Can you work these out from the model? Positions are in its coordinate system, mm. A direction names the side the tool comes from. Round coordinates to 2 decimals unless told otherwise and drop trailing zeros. Write each loop counter-clockwise with the first axis right and the second up, starting at its lowest first coordinate (ties: lowest second). Pieces come first, ordered by that corner, then holes. Notation, with made-up numbers: M 38.5,1 L 48.5,1 A33 cw 48.5,36 Z; hole C 74.25,82.25 d4. An arc over 180 degrees is marked long. Answer as a JSON object with one key per item and string values. Group by question number.
1) Suppose I cut it at B-B, the plane y = 19. Write out the boundary of the cut face in (x, z), and give its area (4 significant figures).
2) On a 3-axis mill with a long thin cutter (end or side, diameter ignored), from which of +Z, -Z, +X, -X, +Y, -Y can I reach the whole of each face in a straight line? I mean faces 1 (the flat face through (-1, 13.05, 5)), 2 (the cylindrical face through (9.95, -7.46, 7.71)). Say none if no direction works.
3) Suppose I cut it at A-A, the plane x = 24.9. Write out the boundary of the cut face in (y, z) (3 decimals).
4) If we mould it in two halves opening along Z, with no side actions, what happens to faces 3 (the flat face through (-13, -7, 4.5)), 4 (the cylindrical face through (-4.85, 10.24, 4.59)), 5 (the cylindrical face through (27.76, -7.46, 2.72))? For each: +Z half, -Z half, draft (parallel to the pull), parting line (faces both ways), or undercut.
5) Suppose I cut it at C-C, the plane x = 2.5. Write out the boundary of the cut face in (y, z), and give its area (4 significant figures).
6) Please list where these lines run through material, in increasing order: L1, parallel to Y at x = -23.1, z = 4.5; L2, parallel to X at y = 18, z = 2.25. Write a range as [from, to].
7) I'm going to push flat-ended pins straight in: pin 1 Ø2.5 at (x, y) = (-12.5, -8) entering from +Z; pin 2 Ø1.5 at (x, z) = (13, -0.5) entering from +Y; pin 3 Ø3 at (x, y) = (-2.1, 10.3) entering from +Z. Where does each tip first touch, or does it pass through?
Autodesk Inventor part; units mm, degrees
ref_plane "YZ Plane" through (0, 0, 0) normal (1, 0, 0) x (0, 1, 0)
ref_plane "XZ Plane" through (0, 0, 0) normal (0, 1, 0) x (-1, 0, 0)
ref_plane "XY Plane" through (0, 0, 0) normal (0, 0, 1) x (1, 0, 0)
sketch "Sketch1" plane through (0, 0, 0) normal (0, 0, 1) x (1, 0, 0)
  line L0 (0, 0) -> (-25, 0)
  line L1 (-25, 25) -> (0, 25)
  line L2 (0, 25) -> (0, 0)
  circle A0 centre (-23.1, 22.7984) radius 1.1
  circle A1 centre (-2.1, 22.8) radius 1.1
  circle A2 centre (-23.1, 10.2984) radius 1.1
  circle A3 centre (-2.1, 10.3) radius 1.1
  line L3 (-25, 0) -> (-25.2, 0)
  line L4 (-25.2, 0) -> (-25.2, 25)
  line L5 (-25.2, 25) -> (-25, 25)
  dimension "d2" = 2.2
  dimension "d5" = 2.2
  dimension "d7" = 12.5
  dimension "d8" = 2.2
  dimension "d9" = 2.2
  dimension "d14" = 12.5
  dimension "d31" = 2.1
  dimension "d46" = 0.2
  dimension "d47" = 2.1
  dimension "d48" = 2.1
extrude "Base" add sketch "Sketch1" along normal blind 2
sketch "Sketch2" plane through (0, 0, 2) normal (0, 0, 1) x (1, 0, 0)
  line L0 (-26.5, 0) -> (-26.5, 26.5)
  line L1 (-26.5, 26.5) -> (1.5, 26.5)
  line L2 (1.5, 26.5) -> (1.5, 0)
  line L3 (1.5, 0) -> (0, 0)
  line L4 (0, 25) -> (-25.2, 25)
  line L5 (0, 0) -> (0, 25)
  line L6 (-25.2, 25) -> (-25.2, 0)
  line L7 (-25.2, 0) -> (-26.5, 0)
  point P0 (-25, 25)
  point P1 (-25, 0)
  dimension "d16" = 26.5
  dimension "d17" = 28
extrude "Walls" add sketch "Sketch2" along normal blind 5.25 and the other way blind 2
sketch "Sketch3" plane through (0, 0, 2) normal (0, 0, 1) x (1, 0, 0)
  circle A0 centre (-23.1, 10.2984) radius 1.1
  circle A1 centre (-23.1, 10.2984) radius 1.6
  circle A2 centre (-2.1, 10.3) radius 1.1
  circle A3 centre (-2.1, 10.3) radius 1.6
  circle A4 centre (-23.1, 22.7984) radius 1.1
  circle A5 centre (-23.1, 22.7984) radius 1.6
  circle A6 centre (-2.1, 22.8) radius 1.1
  circle A7 centre (-2.1, 22.8) radius 1.6
  point P0 (0, 0)
  dimension "d22" = 3.2
  dimension "d23" = 3.2
  dimension "d24" = 3.2
  dimension "d25" = 3.2
extrude "Spacers" add sketch "Sketch3" along normal up to surface (5.25 mm away)
sketch "Sketch4" plane through (0, 0, 2) normal (0, 0, 1) x (1, 0, 0)
  circle A0 centre (-23.1, 10.2984) radius 1.1
  arc A1 (-23.1938, 7.55) -> (-23.1, 13.0484) centre (-23.1, 10.2984) ccw
  circle A2 centre (-2.1, 10.3) radius 1.1
  arc A3 (-2.1, 13.05) -> (-2.1, 7.55) centre (-2.1, 10.3) ccw
  circle A4 centre (-23.1, 22.7984) radius 1.1
  circle A5 centre (-2.1, 22.8) radius 1.1
  line L0 (-4.85, 22.8) -> (-4.85, 25)
  line L1 (-25.2, 25) -> (0, 25)
  line L2 (-2.1, 20.05) -> (0, 20.05)
  line L3 (0, 25) -> (0, 0)
  line L4 (-2.1, 13.05) -> (0, 13.05)
  line L5 (-2.1, 7.55) -> (0, 7.55)
  line L6 (-23.1, 13.0484) -> (-25.2, 13.0484)
  line L7 (-23.1938, 7.55) -> (-25, 7.55)
  arc A6 (-4.85, 22.8) -> (-2.1, 20.05) centre (-2.1, 22.8) ccw
  line L8 (-25, 7.55) -> (-25.2, 7.55)
  line L9 (-25.2, 13.0484) -> (-25.2, 13.0484)
  line L10 (-25.2, 25) -> (-25.2, 0)
  line L11 (-25.2, 20.0484) -> (-25.2, 20.0484)
  line L12 (-20.35, 22.7984) -> (-20.35, 25.6874)
  line L13 (-23.1, 20.0484) -> (-25.85, 20.0484)
  arc A7 (-23.1, 20.0484) -> (-20.35, 22.7984) centre (-23.1, 22.7984) ccw
  point P0 (-25, 25)
  point P1 (-20.35, 25)
  point P2 (-25.2, 20.0484)
  dimension "d33" = 5.5
  dimension "d34" = 5.5
extrude "Spacer blocks" add sketch "Sketch4" along normal up to surface (5.25 mm away)
sketch "Sketch5" plane through (0, 0, 0) normal (0, 0, -1) x (-1, 0, 0)
  line L0 (-1.5, 26.5) -> (-1.5, 0)
  circle A0 centre (12.4, 10.3) radius 4.5
  point P0 (0, 0)
  dimension "d39" = 13.9
  dimension "d40" = 9
extrude "Camera Hole" cut sketch "Sketch5" against normal through all
fillet "Outside Fillet - 2mm" radius 2 1 edges at (-7.9, 10.3, 0)
fillet "Inside Fillet - 1mm" radius 0.5 2 edges at (-7.9, 10.3, 1.9999) (-7.9, 10.3, 2)
chamfer "Chamfer1" distance 0.5 angle 45 5 edges at (1.5, 13.25, 0) (1.5, 26.5, 3.625) (-12.5, 26.5, 0) (-26.5, 26.5, 3.625) (-26.5, 13.25, 0)
sketch "Sketch6" plane through (-25.2, 0, 2) normal (0, -1, 0) x (1, 0, 0)
  line L0 (-0.8, -2) -> (-1.3, -1.5)
  line L1 (26.2, -2) -> (-0.8, -2)
  line L2 (26.7, -1.5) -> (26.2, -2)
  line L3 (26.7, -1.5) -> (26.7, 5.25)
  line L4 (25.2, 5.25) -> (26.7, 5.25)
  line L5 (25.2, 0) -> (25.2, 5.25)
  line L6 (0, 0) -> (25.2, 0)
  line L7 (0, 0) -> (0, 5.25)
  line L8 (-1.3, 5.25) -> (0, 5.25)
  line L9 (-1.3, -1.5) -> (-1.3, 5.25)
  point P0 (25.2, -2)
extrude "Bottom Extension" add sketch "Sketch6" along normal blind 5
sketch "Sketch7" plane through (-25.2, -5, 2) normal (0, -1, 0) x (1, 0, 0)
  line L0 (26.7, 5.25) -> (25.2, 5.25)
  line L1 (26.7, 5.25) -> (20.1, 5.25)
  line L2 (20.1, 5.25) -> (20.1, -2)
  line L3 (20.1, -2) -> (50.1, -2)
  line L4 (50.1, -2) -> (50.1, 5.25)
  line L5 (50.1, 5.25) -> (26.7, 5.25)
  line L6 (26.7, 5.25) -> (25.2, 5.25) construction
  line L7 (25.2, 5.25) -> (25.2, 0) construction
  line L8 (25.2, 0) -> (0, 0) construction
  line L9 (0, 0) -> (0, 5.25) construction
  line L10 (0, 5.25) -> (-1.3, 5.25) construction
  line L11 (-1.3, 5.25) -> (-1.3, -1.5) construction
  line L12 (-1.3, -1.5) -> (-0.8, -2) construction
  line L13 (-0.8, -2) -> (26.2, -2) construction
  line L14 (26.2, -2) -> (26.7, -1.5) construction
  line L15 (26.7, -1.5) -> (26.7, 5.25) construction
  line L16 (20.1, -2) -> (-0.8, -2)
  line L17 (-1.3, -1.5) -> (-0.8, -2)
  line L18 (-1.3, -1.5) -> (-1.3, 5.25)
  line L19 (-1.3, 5.25) -> (0, 5.25)
  line L20 (0, 5.25) -> (5.1, 5.25)
  line L21 (5.1, 5.25) -> (5.1, 0)
  line L22 (5.1, 0) -> (20.1, 0)
  line L23 (5.1, 0) -> (5.1, 2.5)
  line L24 (5.1, 2.5) -> (20.1, 2.5)
  point P0 (25.2, -2)
  dimension "d54" = 6.6
  dimension "d55" = 30
  dimension "d58" = 5.1
  dimension "d59" = 2.5
extrude "Mounting Arm" add sketch "Sketch7" along normal blind 5
sketch "Sketch8" plane through (-25.2, -5, 2) normal (0, 1, 0) x (1, 0, 0)
  line L0 (50.1, 2) -> (50.1, -5.25)
  circle A0 centre (50.1, -1.625) radius 15
  point P0 (25.2, 2)
  dimension "d60" = 30
extrude "Mounting Disk" add sketch "Sketch8" against normal up to surface (5 mm away)
fillet "Fillet4" radius 2.5 2 edges at (10.3446, -7.5, 0) (10.3446, -7.5, 7.25)
sketch "Sketch9" plane through (-25.2, -5, 2) normal (0, 1, 0) x (1, 0, 0)
  arc A0 (36.0488, -6.875) -> (36.0488, 3.625) centre (50.1, -1.625) ccw
  circle A1 centre (50.1, -1.625) radius 3
  point P0 (25.2, 2)
  dimension "d64" = 6
extrude "Center Hole" cut sketch "Sketch9" against normal through all
properties part number "Top L"
Results:
{
 "1": {"outline": "M -26.5,0.5 L -26,0 L 1,0 L 1.5,0.5 L 1.5,7.25 L 0,7.25 L 0,2 L -25.2,2 L -25.2,7.25 L -26.5,7.25 Z", "area": "70.45 mm^2"},
 "2": {"face 1": "+Z", "face 2": "+Z, -X, +Y, -Y"},
 "3": {"outline": "M -10,-11.375 L -5,-11.375 L -5,0.625 L -10,0.625 Z; M -10,6.625 L -5,6.625 L -5,18.625 L -10,18.625 Z"},
 "4": {"face 3": "+Z half", "face 4": "draft", "face 5": "undercut"},
 "5": {"outline": "M -10,0 L -5,0 L -5,7.25 L -10,7.25 Z", "area": "36.25 mm^2"},
 "6": {"L1": "[-10, -5], [7.55, 9.2], [11.4, 13.05], [20.05, 21.7], [23.9, 26.5]", "L2": "[-26.5, -25.2], [0, 1.5]"},
 "7": {"pin 1": "z = 4.5", "pin 2": "y = -5", "pin 3": "z = 7.25"}
}
